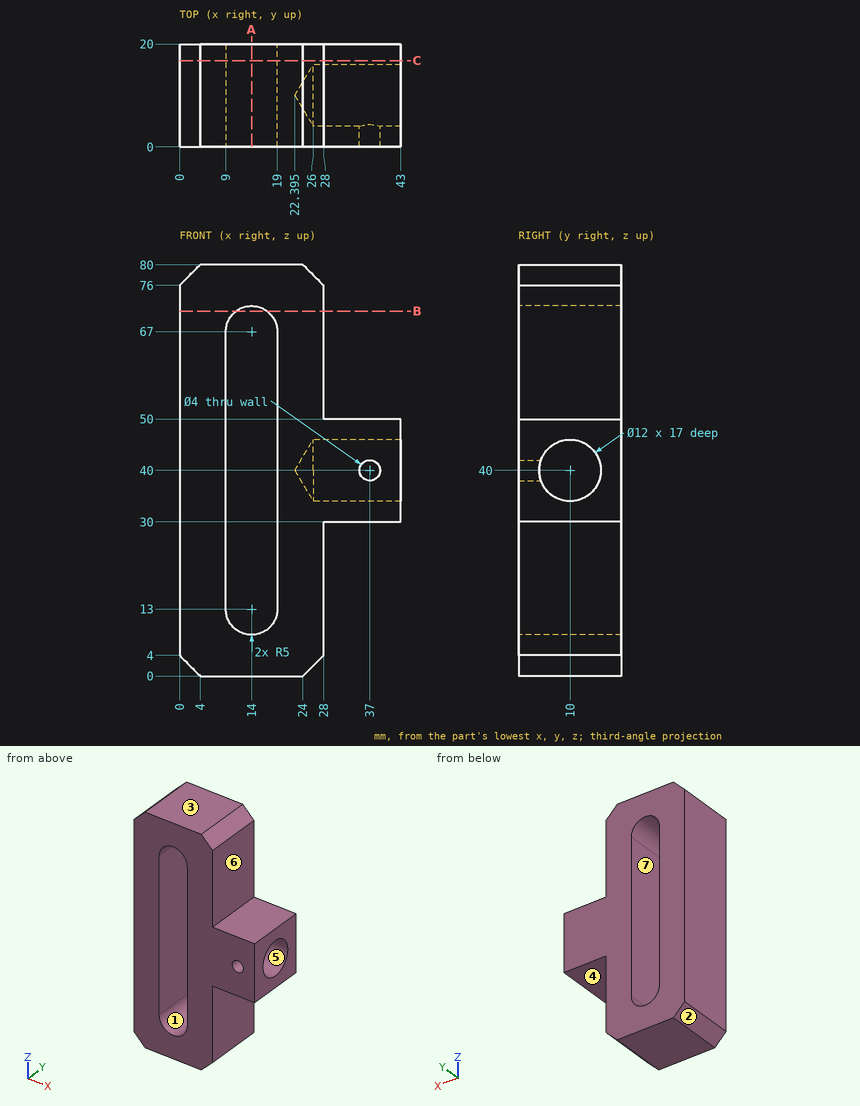
Geometry check sheet. Reference: drawing and pictorial views, mm from the part's lowest x, y, z. A direction names the side the tool comes from. Give positions to 0.01 mm unless a question says otherwise; leave off trailing zeros. Write each loop counter-clockwise with the first axis right and the second up, starting at its lowest first coordinate (ties: lowest second). Pieces come first, ordered by that corner, then holes. Notation, with made-up numbers: (19, -20) -> (64, -20) arc R27 cw to (64, 16) -> close; hole circle Ø4 at (-9.75, 82). An arc over 180 degrees is marked (long way). One line per item, written item: value. Start each with the question number.
Item 1: Draft check along Z on the marked faces 1, 2 and 3. Enter one of: +Z half, -Z half, draft (parallel to the pull), parting line (faces both ways), or undercut.
Item 2: Gauge pin test, flat ends, axial feed: pin 1 (12 mm diameter, centred on x = 32.5, y = 5.5, fed in from -Z); pin 2 (6 mm diameter, centred on y = 13, z = 59, fed in from +X); pin 3 (6 mm diameter, centred on y = 11, z = 51, fed in from +X); pin 4 (3 mm diameter, centred on x = 37, z = 40, fed in from -Y). Record the tip position at first contact, or that the pin passes through.
Item 3: Section check A-A on x = 14. Record the cut outline in (y, z), then the cut area to 3 significant figures.
Item 4: Tool access check on the marked faces 4, 5, 6 and 7. Record the directions out of +Z, -Z, +X, -X, +Y, -Y that give a thin tool (end or side, any length) a straight path to the whole face; none if there is none.
Item 5: Section check B-B on z = 71. Record the cut outline in (x, y).
Item 6: Section check C-C on y = 16.75. Record the cut outline in (x, z).
Item 7: Material ranges on probe 1 along X at (y, z) = (4.5, 17.5); probe 2 along Z at (x, y) = (32.5, 10); probe 3 along Z at (x, y) = (37, 2.5), recorded low to high. Write a range as from..to.
Results list:
1. face 1: undercut
1. face 2: -Z half
1. face 3: +Z half
2. pin 1: z = 2.5
2. pin 2: x = 28
2. pin 3: x = 43
2. pin 4: y = 15.81
3. outline: (0, 0) -> (20, 0) -> (20, 8) -> (0, 8) -> close; (0, 72) -> (20, 72) -> (20, 80) -> (0, 80) -> close
3. area: 320 mm²
4. face 4: -Z, +X, +Y, -Y
4. face 5: +X
4. face 6: +Z, +X, +Y, -Y
4. face 7: +Y, -Y
5. outline: (0, 0) -> (11, 0) -> (11, 20) -> (0, 20) -> close; (17, 0) -> (28, 0) -> (28, 20) -> (17, 20) -> close
6. outline: (0, 4) -> (4, 0) -> (24, 0) -> (28, 4) -> (28, 30) -> (43, 30) -> (43, 50) -> (28, 50) -> (28, 76) -> (24, 80) -> (4, 80) -> (0, 76) -> close; hole (9, 13) arc R5 ccw to (19, 13) -> (19, 67) arc R5 ccw to (9, 67) -> close
7. probe 1: 0..9, 19..28
7. probe 2: 30..34, 46..50
7. probe 3: 30..38, 42..50
